```python
from build123d import *

# Parameters (mm, degrees)
SKETCH1_R           = 4
BOSS_EXTRUDE1_DEPTH = 9.25
SKETCH2_R           = 4
BOSS_EXTRUDE2_DEPTH = 1
SKETCH3_R           = 4
SKETCH3_R_2         = 2.45
BOSS_EXTRUDE3_DEPTH = 5.6
SKETCH5_R           = 6
BOSS_EXTRUDE4_DEPTH = 2
FILLET1_R           = 1


with BuildPart() as part:
    # Sketch1 → Boss-Extrude1 (new body)
    with BuildSketch(Plane(origin=(0, 0, 0), x_dir=(1, 0, 0), z_dir=(0, 1, 0))):
        Circle(SKETCH1_R)
        with BuildLine():
            Line((-1.12, 1.170469991), (1.12, 1.170469991))
            ThreePointArc((1.12, 1.170469991), (0, -1.62), (-1.12, 1.170469991))
        make_face(mode=Mode.SUBTRACT)
    extrude(amount=BOSS_EXTRUDE1_DEPTH)

    # Sketch2 → Boss-Extrude2 (add)
    with BuildSketch(Plane(origin=(0, 9.25, 0), x_dir=(1, 0, 0), z_dir=(0, 1, 0))):
        Circle(SKETCH2_R)
    extrude(amount=BOSS_EXTRUDE2_DEPTH)

    # Sketch3 → Boss-Extrude3 (add)
    with BuildSketch(Plane(origin=(0, 10.25, 0), x_dir=(1, 0, 0), z_dir=(0, 1, 0))):
        Circle(SKETCH3_R)
        Circle(SKETCH3_R_2, mode=Mode.SUBTRACT)
    extrude(amount=BOSS_EXTRUDE3_DEPTH)

    # Sketch5 → Boss-Extrude4 (add)
    with BuildSketch(Plane(origin=(0, 2.25, 0), x_dir=(1, 0, 0), z_dir=(0, 1, 0))):
        Circle(SKETCH5_R)
        with BuildLine():
            Line((1.12, 1.170469991), (-1.12, 1.170469991))
            ThreePointArc((-1.12, 1.170469991), (0, -1.62), (1.12, 1.170469991))
        make_face(mode=Mode.SUBTRACT)
    extrude(amount=BOSS_EXTRUDE4_DEPTH)

    # Fillet1
    fillet1_edges = [part.edges().sort_by_distance(p)[0] for p in [
        (-4, 4.25, 0),
    ]]
    fillet(fillet1_edges, radius=FILLET1_R)


solid = part.part
```
Geometry check sheet. Reference: the model listing, model coordinates, mm. A direction names the side the tool comes from. Coordinates: 2 decimals unless noted, no trailing zeros. Loops run counter-clockwise (first coordinate to the right, second up) from the corner with the lowest first, then second, coordinate; pieces in that order, holes last. Notation, with made-up numbers: (66.5, 80.25) - (123.5, 80.25) arc R20 ccw to (123.5, 112.25) - close; hole circle Ø11 at (-29, 3.25). An arc over 180 degrees is marked (long way). One line per item, written item: value. Start each with the question number.
(1) Tool access check on faces 1 (the cylindrical face through (-0.867, 1.109, 3.905)), 2 (the cylindrical face through (-0.5, 13, 2.4)), 3 (the flat face through (2, 0, 0)). Record the directions out of +Z, -Z, +X, -X, +Y, -Y that give a thin tool (end or side, any length) a straight path to the whole face; none if there is none.
(2) Material ranges on line 1 (X direction, y = 14.6, z = 0); line 2 (Y direction, x = 1.5, z = -1.25), recorded low to high. Write a range as [from, to].
(3) Cross-section at B-B on z = 0. Enter the section's corners in (x, y), plus the area to 3 significant figures.
(4) Cross-section at A-A on x = 0. Enter the section's corners in (y, z), plus the area to 3 significant figures.
(5) Mould release check, pull along X, two halves, no side actions. Record for faces 4 (the cylindrical face through (-6, 3, 0)), 5 (the flat face through (-4, 4.25, -4)), 6 (the flat face through (0, 5, -1.17)): released by +X, released by -X, zero draft, split by the parting line, or undercut.
(6) Cross-section at C-C on y = 12.25. Enter the section's corners in (x, z), plus the area to 3 significant figures.
(7) Cross-section at D-D on y = 1.75. Enter the section's corners in (x, z).
(8) Depth check by flat-ended pin: P1, Ø1, axis at x = -3.5, y = 4.5, coming from the +Z side; P2, Ø2, axis at y = 13, z = 1, coming from the -X side; P3, Ø5, axis at x = 4.5, y = 4, coming from the -Z side. Enter the tip coordinate at first touch or a pass-through.
Results below:
1. face 1: -Y
1. face 2: +Y
1. face 3: +Z, -Z, +X, -X, -Y
2. line 1: x = [-4, -2.45], [2.45, 4]
2. line 2: y = [0, 10.25]
3. outline: (-6, 2.25) - (-4, 2.25) - (-4, 0) - (-1.62, 0) - (-1.62, 9.25) - (1.62, 9.25) - (1.62, 0) - (4, 0) - (4, 2.25) - (6, 2.25) - (6, 4.25) - (5, 4.25) arc R1 cw to (4, 5.25) - (4, 15.85) - (2.45, 15.85) - (2.45, 10.25) - (-2.45, 10.25) - (-2.45, 15.85) - (-4, 15.85) - (-4, 5.25) arc R1 cw to (-5, 4.25) - (-6, 4.25) - close
3. area: 77.8 mm2
4. outline: (0, -4) - (2.25, -4) - (2.25, -6) - (4.25, -6) - (4.25, -5) arc R1 cw to (5.25, -4) - (15.85, -4) - (15.85, -2.45) - (10.25, -2.45) - (10.25, 2.45) - (15.85, 2.45) - (15.85, 4) - (5.25, 4) arc R1 cw to (4.25, 5) - (4.25, 6) - (2.25, 6) - (2.25, 4) - (0, 4) - (0, 1.62) - (9.25, 1.62) - (9.25, -1.17) - (0, -1.17) - close
4. area: 82.0 mm2
5. face 4: split by the parting line
5. face 5: zero draft
5. face 6: undercut
6. outline: circle Ø8 at (0, 0); hole circle Ø4.9 at (0, 0)
6. area: 31.4 mm2
7. outline: circle Ø8 at (0, 0); hole (-1.12, -1.17) - (1.12, -1.17) arc R1.62 ccw (long way) to start
8. P1: stops at z = 5.16
8. P2: stops at x = -4
8. P3: stops at z = -5.66
